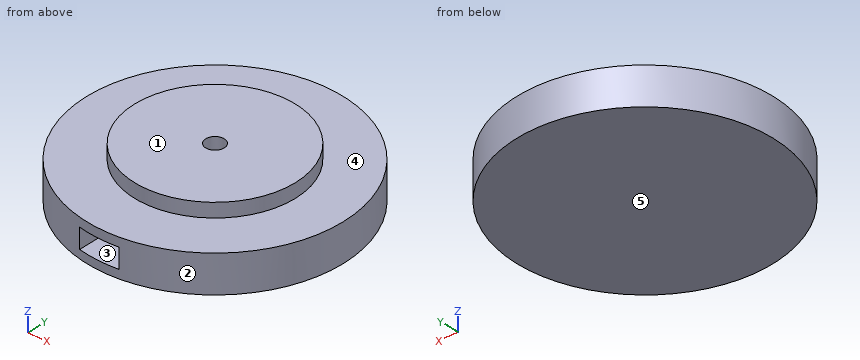
```python
from build123d import *

# Parameters (mm, degrees)
F0_R      = 27.5
F1_DEPTH  = 8
F2_R      = 17.25
F3_DEPTH  = 3
F4_W      = 10.243726
F4_H      = 7.44366
F5_DEPTH  = 7
F6_W      = 8.55
F6_H      = 4.25
F7_DEPTH  = 25
F8_R      = 2
F9_DEPTH  = 25
F10_W     = 10.243726
F10_H     = 7.44366
F11_DEPTH = 1


with BuildPart() as f1:
    # F0 (on Top) → F1 (new body)
    with BuildSketch(Plane.XY):
        Circle(F0_R)
    extrude(amount=F1_DEPTH)

    # F2 (on face) → F3 (join)
    with BuildSketch(Plane.XY.offset(8)):
        Circle(F2_R)
    extrude(amount=F3_DEPTH)

    # F4 (on face) → F5 (cut)
    with BuildSketch(Plane(origin=(0, 0, 0), x_dir=(1, 0, 0), z_dir=(0, 0, -1))):
        with Locations((-0.102693, 0.080894)):
            Rectangle(F4_W, F4_H)
    extrude(amount=-F5_DEPTH, mode=Mode.SUBTRACT)

    # F6 (on face) → F7 (cut)
    with BuildSketch(Plane(origin=(0, -3.802724, 0), x_dir=(-1, 0, 0), z_dir=(0, 1, 0))):
        with Locations((0.52315, 3.955042)):
            Rectangle(F6_W, F6_H)
    extrude(amount=-F7_DEPTH, mode=Mode.SUBTRACT)

    # F8 (on face) → F9 (cut)
    with BuildSketch(Plane(origin=(0, 0, 7), x_dir=(1, 0, 0), z_dir=(0, 0, -1))):
        Circle(F8_R)
    extrude(amount=-F9_DEPTH, mode=Mode.SUBTRACT)

    # F10 (on face) → F11 (join)
    with BuildSketch(Plane(origin=(0, 0, 0), x_dir=(1, 0, 0), z_dir=(0, 0, -1))):
        with Locations((-0.102693, 0.080894)):
            Rectangle(F10_W, F10_H)
    extrude(amount=-F11_DEPTH)


solid = f1.part
```
Input: part model. Units: mm. Frame: model coordinates. Face numbers are marked on the shaded views. A direction names the side the tool comes from. Coordinates: 2 decimals unless noted, no trailing zeros. Write each loop counter-clockwise with the first axis right and the second up, starting at its lowest first coordinate (ties: lowest second). Pieces come first, ordered by that corner, then holes. Notation, with made-up numbers: (-40, 18) -> (16, 18) arc R23 cw to (16, 33) -> close; hole circle Ø7 at (-22.75, 31.25). An arc over 180 degrees is marked (long way). Answer as a JSON object with one key per item and string values.
1. Access query for the marked faces 4 and 5. Directions: +Z, -Z, +X, -X, +Y, -Y. A direction counts if a zero-diameter tool reaches every point of the face in a straight line with its end or side. Return the directions, or none.
Result set:
{"face 4": "+Z", "face 5": "-Z, +X, -X, +Y, -Y"}
2. Section A-A on x = 0. Return the cut outline in (y, z).
Result set:
{"outline": "(-27.5, 0) -> (27.5, 0) -> (27.5, 8) -> (17.25, 8) -> (17.25, 11) -> (2, 11) -> (2, 7) -> (3.64, 7) -> (3.64, 1) -> (-3.8, 1) -> (-3.8, 1.83) -> (-27.5, 1.83) -> close; (-27.5, 6.08) -> (-3.8, 6.08) -> (-3.8, 7) -> (-2, 7) -> (-2, 11) -> (-17.25, 11) -> (-17.25, 8) -> (-27.5, 8) -> close"}
3. Section D-D on x = 11. Return the cut outline in (y, z).
Result set:
{"outline": "(-25.2, 0) -> (25.2, 0) -> (25.2, 8) -> (13.29, 8) -> (13.29, 11) -> (-13.29, 11) -> (-13.29, 8) -> (-25.2, 8) -> close"}
4. Material intervals for line 1 (Y direction, x = 0, z = 8.6); line 2 (Z direction, x = -4, y = -8.5); line 3 (Z direction, x = 25, y = 7.5), sorted ascending. Write a range as from..to.
Result set:
{"line 1": "y = -17.25..-2, 2..17.25", "line 2": "z = 0..1.83, 6.08..11", "line 3": "z = 0..8"}
5. Section B-B on y = -10.5. Return the cut outline in (x, z).
Result set:
{"outline": "(-25.42, 0) -> (25.42, 0) -> (25.42, 8) -> (13.69, 8) -> (13.69, 11) -> (-13.69, 11) -> (-13.69, 8) -> (-25.42, 8) -> close; hole (-4.8, 1.83) -> (3.75, 1.83) -> (3.75, 6.08) -> (-4.8, 6.08) -> close"}
6. First-contact query: P1, Ø6, axis at x = -1, z = 5.5, coming from the +Y side; P2, Ø3, axis at y = -0.5, z = 3.5, coming from the +X side; P3, Ø2, axis at y = -18, z = 4.5, coming from the -X side; P4, Ø3.5, axis at x = 0, y = 0, coming from the +Z side. Flat tips, straight axial feed; report the tip coordinate or a pass-through.
Result set:
{"P1": "stops at y = 27.5", "P2": "stops at x = 27.5", "P3": "stops at x = -21.62", "P4": "stops at z = 1"}
7. Section C-C on y = 0. Return the cut outline in (x, z).
Result set:
{"outline": "(-27.5, 0) -> (27.5, 0) -> (27.5, 8) -> (17.25, 8) -> (17.25, 11) -> (2, 11) -> (2, 7) -> (5.02, 7) -> (5.02, 1) -> (-5.22, 1) -> (-5.22, 7) -> (-2, 7) -> (-2, 11) -> (-17.25, 11) -> (-17.25, 8) -> (-27.5, 8) -> close"}
8. Mould query, pull axis X, two halves, no side actions, for the marked faces 1, 2 and 3. Classes: released by +X, released by -X, zero draft, split by the parting line, or undercut.
Result set:
{"face 1": "zero draft", "face 2": "split by the parting line", "face 3": "undercut"}
